Build history of the part. All positions in model axes, mm. Face numbers are marked on the shaded views. Coordinates: 2 decimals unless noted, no trailing zeros. Order: outer loops, then holes, each group sorted by start corner. A loop starts at its lowest first (then second) coordinate and runs counter-clockwise, first axis right, second up. Notation, with made-up numbers: (21, 12) - (46, 12) arc R29 cw to (46, 46) - close; hole circle Ø9 at (-34, 17.25). An arc over 180 degrees is marked (long way). Write each question's results on one line, items separated by ' | '.
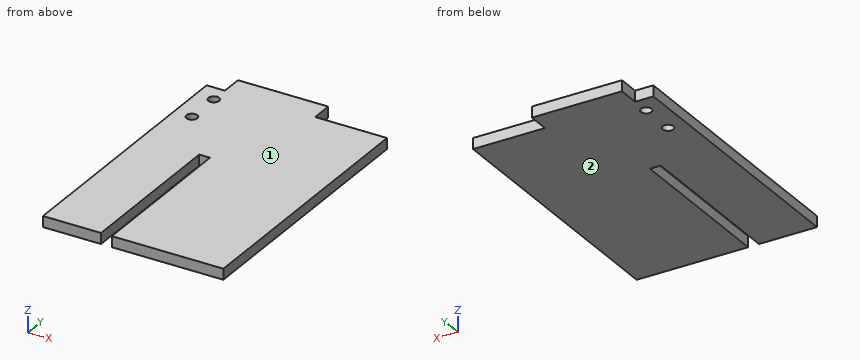
from build123d import *

# Parameters (mm, degrees)
BOSS_EXTRUDE1_DEPTH = 3
SKETCH2_R           = 1.5
CUT_EXTRUDE1_DEPTH  = 4


with BuildPart() as part:
    # Sketch1 → Boss-Extrude1 (new body)
    with BuildSketch(Plane.XY):
        Polygon((12.5, 73.857731997), (-12.5, 73.857731997), (-12.5, 67.857731997), (-17.58, 67.857731997), (-17.58, -7.142268003), (-1.5, -7.142268003), (-1.5, 37.857731997), (1.5, 37.857731997), (1.5, -7.142268003), (32.42, -7.142268003), (32.42, 67.857731997), (12.5, 67.857731997), align=None)
    extrude(amount=BOSS_EXTRUDE1_DEPTH)

    # Sketch2 → Cut-Extrude1 (cut, through all)
    with BuildSketch(Plane.XY.offset(3)):
        with Locations((-12.58, 62.857731997)):
            Circle(SKETCH2_R)
        with Locations((-12.58, 52.857731997)):
            Circle(SKETCH2_R)
    extrude(amount=-CUT_EXTRUDE1_DEPTH, mode=Mode.SUBTRACT)


solid = part.part
1. Drop flat-ended pins along their axis: pin 1 Ø2.5 at (x, y) = (-12.58, 52.86) entering from +Z; pin 2 Ø0.9 at (x, z) = (23, 1.5) entering from +Y. Give the stop position or say it passes through.
Solved:
pin 1: passes through | pin 2: stops at y = 67.86
2. Band-saw the part on A-A on y = 8. Give the cut face in (x, z).
Solved:
outline: (-17.58, 0) - (-1.5, 0) - (-1.5, 3) - (-17.58, 3) - close; (1.5, 0) - (32.42, 0) - (32.42, 3) - (1.5, 3) - close
3. Band-saw the part on C-C on z = 1. Give the cut face in (x, y), then the cut area to 3 significant figures.
Solved:
outline: (-17.58, -7.14) - (-1.5, -7.14) - (-1.5, 37.86) - (1.5, 37.86) - (1.5, -7.14) - (32.42, -7.14) - (32.42, 67.86) - (12.5, 67.86) - (12.5, 73.86) - (-12.5, 73.86) - (-12.5, 67.86) - (-17.58, 67.86) - close; hole circle Ø3 at (-12.58, 52.86); hole circle Ø3 at (-12.58, 62.86) | area: 3,750 mm2
4. Band-saw the part on B-B on x = 14. Give the cut face in (y, z).
Solved:
outline: (-7.14, 0) - (67.86, 0) - (67.86, 3) - (-7.14, 3) - close
5. Probe line 1 (Y direction, x = -12.58, z = 1.5); line 2 (X direction, y = 8, z = 1.4); line 3 (Y direction, x = 29, z = 0.35). List the from-to ranges inside material, lowest first.
Solved:
line 1: y = -7.14 to 51.36, 54.36 to 61.36, 64.36 to 67.86 | line 2: x = -17.58 to -1.5, 1.5 to 32.42 | line 3: y = -7.14 to 67.86
6. Two-plate mould, pull along Z, no slides. Class the marked faces 1 and 2: +Z half, -Z half, draft (parallel to the pull), parting line (faces both ways), or undercut.
Solved:
face 1: +Z half | face 2: -Z half
